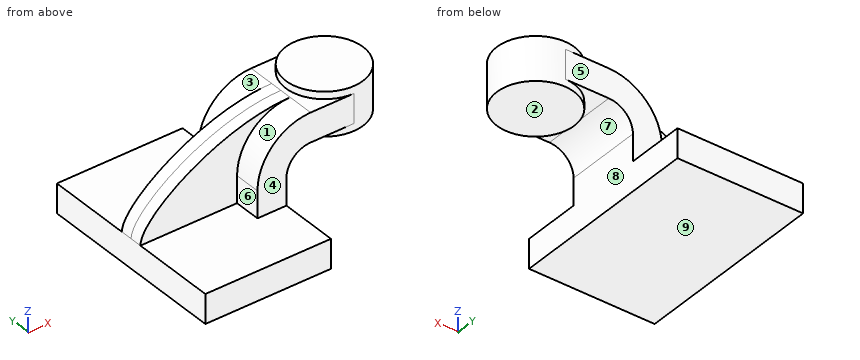
from build123d import *

# Parameters (mm, degrees)
F1_DEPTH = 63.5
F0_W     = 25.4
F0_H     = 19.05
F2_DEPTH = 25.4
F3_DEPTH = 7.9375


with BuildPart() as f1:
    # F0 (on Front) → F1 (new body, symmetric)
    with BuildSketch(Plane.XZ):
        Polygon((41.275, -9.525), (41.275, 9.525), (22.225, 9.525), (-41.275, 9.525), (-41.275, -9.525), align=None)
    extrude(amount=F1_DEPTH, both=True)

    # F0 (on Front) → F2 (join, symmetric)
    with BuildSketch(Plane.XZ):
        with BuildLine():
            Line((22.225, 9.525), (41.275, 9.525))
            Line((41.275, 9.525), (41.275, 27.0002))
            ThreePointArc((41.275, 27.0002), (45.9246798487, 38.2255201513), (57.15, 42.8752))
            Line((57.15, 42.8752), (60.325, 42.8752))
            Line((60.325, 42.8752), (60.325, 61.9252))
            Line((60.325, 61.9252), (57.15, 61.9252))
            ThreePointArc((57.15, 61.9252), (32.4542956671, 51.6959043329), (22.225, 27.0002))
            Line((22.225, 27.0002), (22.225, 9.525))
        make_face()
        with Locations((73.025, 52.4002)):
            Rectangle(F0_W, F0_H)
    extrude(amount=F2_DEPTH, both=True)

    # F0 (on Front) → F3 (join, symmetric)
    with BuildSketch(Plane.XZ):
        with BuildLine():
            Line((-41.275, 9.525), (22.225, 9.525))
            Line((22.225, 9.525), (22.225, 27.0002))
            ThreePointArc((22.225, 27.0002), (32.4542956671, 51.6959043329), (57.15, 61.9252))
            add(Edge.make_bspline(
                [(-41.275, 9.525), (-41.1306880414, 26.5983454883), (10.3886332363, 62.302429229), (57.15, 61.9252)],
                knots=[0, 0, 0, 0, 111.5045361635, 111.5045361635, 111.5045361635, 111.5045361635], degree=3))
        make_face()
    extrude(amount=F3_DEPTH, both=True)

    # F0 (on Front) → F4 (revolve)
    with BuildSketch(Plane.XZ):
        Polygon((85.725, 61.9252), (85.725, 42.8752), (85.725, 38.1), (111.125, 38.1), (111.125, 66.675), (85.725, 66.675), align=None)
    revolve(axis=Axis((85.725, 0, 52.3875), (0, 0, -1)))


solid = f1.part
The model under review builds one solid part; all positions refer to its coordinate system, in mm. Face numbers are marked on the shaded views. A direction names the side the tool comes from. Round coordinates to 2 decimals unless told otherwise and drop trailing zeros. Write each loop counter-clockwise with the first axis right and the second up, starting at its lowest first coordinate (ties: lowest second). Pieces come first, ordered by that corner, then holes. Notation, with made-up numbers: (34, 17) -> (39, 17) arc R27 cw to (39, 36) -> close; hole circle Ø5 at (40, 6). An arc over 180 degrees is marked (long way). Answer as a JSON object with one key per item and string values.
1. We need section C-C on x = 99.5. State the section outline as (y, z) points (3 decimals), and give its area (3 significant figures).
Results found:
{"outline": "(-21.34, 38.1) -> (21.34, 38.1) -> (21.34, 66.675) -> (-21.34, 66.675) -> close", "area": "1,220 mm^2"}
2. Clearance check with flat-ended pins moving along their axes: pin 1 (10 mm diameter, centred on y = 22, z = 34, fed in from -X); pin 2 (10 mm diameter, centred on x = 67.5, z = 35, fed in from +Y); pin 3 (15.5 mm diameter, centred on x = 49.5, z = 41, fed in from +Y); pin 4 (14 mm diameter, centred on y = 20, z = 15.5, fed in from -X) (3 decimals). State where each tip first meets the part, or that it passes through.
Results found:
{"pin 1": "stops at x = 22.28", "pin 2": "stops at y = 20.99", "pin 3": "stops at y = 25.4", "pin 4": "stops at x = -41.275"}
3. We need section A-A on y = 56. State the section outline as (x, z) points (3 decimals).
Results found:
{"outline": "(-41.275, -9.525) -> (41.275, -9.525) -> (41.275, 9.525) -> (-41.275, 9.525) -> close"}
4. Machinability: for the marked faces 1, 2, 3, 4 and 5, which of the approach directions +Z, -Z, +X, -X, +Y, -Y give a long, thin tool a straight path to every point of the face, cutting with its end or side? Answer none if there is none.
Results found:
{"face 1": "+Z, -X, -Y", "face 2": "-Z, +X, +Y, -Y", "face 3": "+Z, -X, +Y", "face 4": "+Z, +X, -X, -Y", "face 5": "+Z, +X, -X, +Y"}
5. The part is to be moulded in two halves that separate along X. For the marked faces 6, 7, 8 and 9, say which applies: pulls with the +X half, pulls with the -X half, needs draft (parallel to the pull), parting line crosses it, or undercut.
Results found:
{"face 6": "pulls with the -X half", "face 7": "undercut", "face 8": "pulls with the +X half", "face 9": "needs draft"}
6. To check wall thickness, follow line 1 along Y through (x, z) = (86, 57.5); line 2 along Z through (x, y) = (-33.5, -40) (3 decimals); line 3 along Z through (x, y) = (82.5, -17.5) (3 decimals). State the ranges of each line that lie inside material, in increasing order.
Results found:
{"line 1": "y = -25.4 to 25.4", "line 2": "z = -9.525 to 9.525", "line 3": "z = 38.1 to 66.675"}
7. We need section B-B on x = 79. State the section outline as (y, z) points (3 decimals), and give its area (3 significant figures).
Results found:
{"outline": "(-25.4, 42.875) -> (-24.494, 42.875) -> (-24.494, 38.1) -> (24.494, 38.1) -> (24.494, 42.875) -> (25.4, 42.875) -> (25.4, 61.925) -> (24.494, 61.925) -> (24.494, 66.675) -> (-24.494, 66.675) -> (-24.494, 61.925) -> (-25.4, 61.925) -> close", "area": "1,430 mm^2"}
